Build history of the part. All positions in model axes, mm. A direction names the side the tool comes from. Give positions to 0.01 mm unless a question says otherwise; leave off trailing zeros. Loops run counter-clockwise (first coordinate to the right, second up) from the corner with the lowest first, then second, coordinate; pieces in that order, holes last.
1) Flat gauge pins, fed straight in: P1, Ø3.5, axis at x = -1.5, y = -2.5, coming from the -Z side; P2, Ø1.5, axis at y = -3.5, z = 227, coming from the +X side; P3, Ø4, axis at y = -3, z = 273.5, coming from the -X side; P4, Ø1.5, axis at y = 3.5, z = 290, coming from the -X side. Where does each tip first touch, or does it go through?
2) Band-saw the part on A-A on z = 337. List the corners of the cut face in (x, y) (3 decimals).
3) 3-axis set-ups, long thin cutter, end or side, ignore diameter. For faces 1 (the cylindrical face through (-1.38, 6.2, 143.62)), 2 (the cylindrical face through (-0.69, -3.1, 340.43)): which of +Z, -Z, +X, -X, +Y, -Y reach the whole face in a straight line?
4) Wall check: line 1 (X direction, y = -1, z = 344); line 2 (Y direction, x = 1.25, z = 82.5); line 3 (Y direction, x = -5.5, z = 234). Give the ranges that are in metal, low to high.
5) Two-plate mould, pull along X, no slides. Class faces 3 (the flat face through (0, -2, 12.7)), 4 (the flat face through (0, 4, 0)), 5 (the conical face through (2.572, -4.033, 304.633)): +X half, -X half, draft (parallel to the pull), parting line (faces both ways), or undercut.
6) Band-saw the part on B-B on z = 118. List the corners of the cut face in (x, y), then the cut area to 3 significant figures.
Solid Edge part; units mm, degrees
sketch "Sketch1" plane through (0, 0, 0) normal (0, 0, 1) x (1, 0, 0)
  circle A0 centre (0, 0) radius 6.35
extrude "Protrusion1" add sketch "Sketch1" along normal blind 365.125
sketch "Sketch2" plane through (0, 0, 0) normal (0, -1, 0) x (1, 0, 0)
  line L0 (6.35, 365.125) -> (6.35, 292.1)
  line L1 (6.35, 292.1) -> (3.175, 317.5)
  line L2 (3.175, 317.5) -> (3.175, 365.125)
  line L3 (3.175, 365.125) -> (6.35, 365.125)
revolve "RevolvedCutout1" cut sketch "Sketch2" angle 360 about axis through (0, 0, 365.125) along (0, 0, -1)
fillet "Round_1" radius 3.175 1 edges at (-3.175, 0, 365.125)
fillet "Round_3" radius 12.7 2 edges at (-3.175, 0, 317.5) (-6.35, 0, 292.1)
sketch "Sketch3" plane through (0.1982, -6.3469, 145.6547) normal (0.0312188, -0.9995126, 0) x (0, 0, -1)
  line L0 (145.6547, 3.175) -> (132.9547, 3.175)
  line L1 (132.9547, 3.175) -> (132.9547, -3.175)
  line L2 (132.9547, -3.175) -> (145.6547, -3.175)
  line L3 (145.6547, -3.175) -> (145.6547, 3.175)
  dimension "D1" = 145.6547
extrude "ExtrudedCutout_1" cut sketch "Sketch3" against normal blind 9.525
hole "Hole_1" at (-3.1735, -0.0991, 6.35) direction (-0.9995126, -0.0312188, 0) diameter 3.175 end up to next
sketch "Sketch4" plane through (-3.1372, -1.2607, 6.35) normal (0.9995126, 0.0312188, 0) x (-0.0312188, 0.9995126, 0)
  circle A0 centre (1.1621, 0) radius 1.5875
extrude "Cutout1" cut sketch "Sketch4" along normal through all
properties material "ABS Plastic, high impact"
Findings below:
1. P1: stops at z = 0
1. P2: stops at x = 5.72
1. P3: stops at x = -6.27
1. P4: stops at x = -5.72
2. outline: circle Ø6.35 at (0, 0)
3. face 1: +Z, -Z
3. face 2: +Z
4. line 1: x = -3.01 to 3.01
4. line 2: y = -6.23 to 6.23
4. line 3: y = -3.17 to 3.17
5. face 3: undercut
5. face 4: draft
5. face 5: parting line
6. outline: circle Ø12.7 at (0, 0)
6. area: 127 mm2
